from build123d import *

# Parameters (mm, degrees)
SKETCH_1_R           = 1.1
EXTRUDE_1_DEPTH      = 5
EXTRUDE_2_DEPTH      = 2.75
EXTRUDE_2_DEPTH_BACK = 7.75
SKETCH_2_W           = 0.5
SKETCH_2_H           = 0.5
SKETCH_3_R           = 0.25
EXTRUDE_3_DEPTH      = 4.5


with BuildPart() as part:
    # Sketch 1 → Extrude 1 (new body)
    with BuildSketch(Plane.XY):
        with Locations(Location((0, 0, 0), (0, 0, 180))):
            Circle(SKETCH_1_R)
    extrude(amount=EXTRUDE_1_DEPTH)

    # Sketch 2 → Extrude 2 (add, two sides: drawn at the far end of the back side and taken through both)
    with BuildSketch(Plane.XY.offset(5).offset(-EXTRUDE_2_DEPTH_BACK)):
        with Locations((-0.000117439, 0)):
            Rectangle(SKETCH_2_W, SKETCH_2_H)
    extrude(amount=EXTRUDE_2_DEPTH + EXTRUDE_2_DEPTH_BACK)

    # Sketch 3 → Extrude 3 (add)
    with BuildSketch(Plane.XZ.offset(0.25)):
        with Locations(Location((0, 7.5, 0), (0, 0, 90))):
            Circle(SKETCH_3_R)
        with Locations(Location((0, -2.5, 0), (0, 0, 270))):
            Circle(SKETCH_3_R)
    extrude(amount=EXTRUDE_3_DEPTH)


solid = part.part
For this review, take the finished solid that the model builds, in its own axes (mm). Give positions to 0.01 mm unless a question says otherwise; leave off trailing zeros. Loops run counter-clockwise (first coordinate to the right, second up) from the corner with the lowest first, then second, coordinate; pieces in that order, holes last. Notation, with made-up numbers: M -37.75,-21.5 L -24.75,-21.5 A32 cw -24.75,10.5 Z; hole C 25,-5.5 d4. An arc over 180 degrees is marked long. Put each result on its own line as item: value. Start each with the question number.
(1) Add section C-C, the plane y = 0. Write out the cut boundary in (x, z).
(2) Add section B-B, the plane z = 0.5. Write out the cut boundary in (x, y).
(3) Add section D-D, the plane x = -0.75. Write out the cut boundary in (y, z).
(4) Wall thickness on L1, parallel to X at y = 0.05, z = 1; L2, parallel to Z at x = -0.85, y = 0; L3, parallel to Y at x = -0.2, z = -0.5: over which ranges is each line inside the solid? List them lowest first.
(5) Add section A-A, the plane y = -3.15. Write out the cut boundary in (x, z), then the cut area to 3 significant figures.
(6) For pin 1 (0.6 mm diameter, centred on x = 0, z = -1, fed in from +Y); pin 2 (0.7 mm diameter, centred on x = 0, y = 0.5, fed in from -Z); pin 3 (0.6 mm diameter, centred on x = 0, z = -1.5, fed in from -Y), all flat-tipped, find the tip position at first contact; note any pin that passes through.
Result:
1. outline: M -1.1,0 L -0.25,0 L -0.25,-2.75 L 0.25,-2.75 L 0.25,0 L 1.1,0 L 1.1,5 L 0.25,5 L 0.25,7.75 L -0.25,7.75 L -0.25,5 L -1.1,5 Z
2. outline: C 0,0 d2.2
3. outline: M -0.8,0 L 0.8,0 L 0.8,5 L -0.8,5 Z
4. L1: x = -1.1 to 1.1
4. L2: z = 0 to 5
4. L3: y = -0.25 to 0.25
5. outline: C 0,-2.5 d0.5; C 0,7.5 d0.5
5. area: 0.393 mm^2
6. pin 1: stops at y = 0.25
6. pin 2: stops at z = -2.75
6. pin 3: stops at y = -0.25
